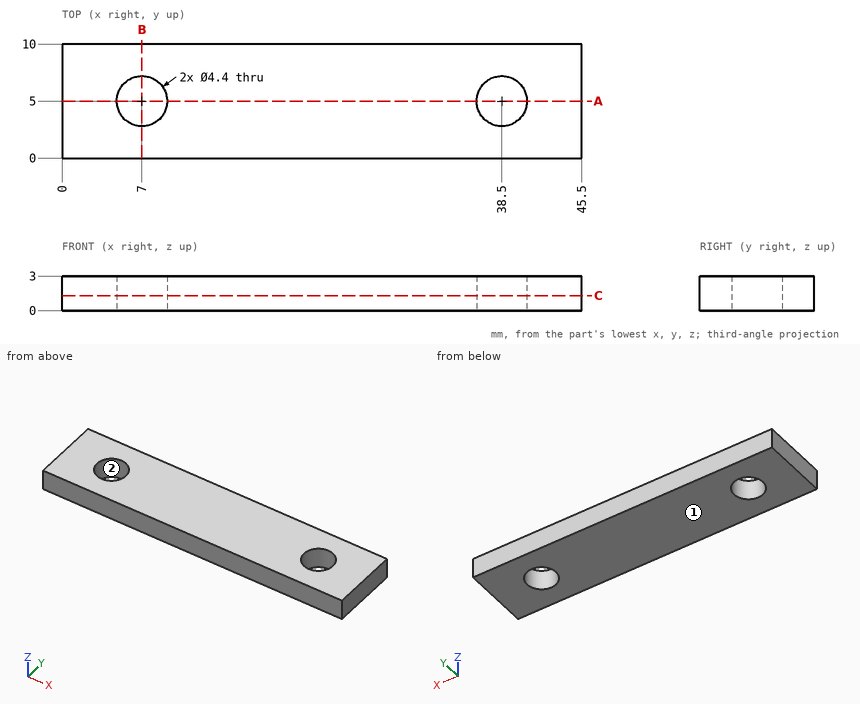
Job drawing, mm, ordinate dimensions from the low corner. One solid piece. Round coordinates to 2 decimals unless told otherwise and drop trailing zeros. Order: outer loops, then holes, each group sorted by start corner. A loop starts at its lowest first (then second) coordinate and runs counter-clockwise, first axis right, second up. Notation, with made-up numbers: (62, 44.25) -> (83, 44.25) arc R35 cw to (83, 78.25) -> close; hole circle Ø2 at (24, -10). An arc over 180 degrees is marked (long way). Write item = value, one per line.
(1) Cut at A-A (y = 5). Write the cut outline in (x, z).
Answers follow:
outline = (0, 0) -> (4.8, 0) -> (4.8, 3) -> (0, 3) -> close; (9.2, 0) -> (36.3, 0) -> (36.3, 3) -> (9.2, 3) -> close; (40.7, 0) -> (45.5, 0) -> (45.5, 3) -> (40.7, 3) -> close
(2) Drill centre lines: L1, parallel to X at y = 5, z = 1.5; L2, parallel to X at y = 7, z = 1.2; L3, parallel to Y at x = 7, z = 2.3. Where is each one in solid material? Low to high.
Answers follow:
L1 = 0 to 4.8, 9.2 to 36.3, 40.7 to 45.5
L2 = 0 to 6.08, 7.92 to 37.58, 39.42 to 45.5
L3 = 0 to 2.8, 7.2 to 10
(3) Pull direction X, two halves, no side cores. Call the marked faces 1 and 2: +X half, -X half, draft (parallel to the pull), parting line (faces both ways), or undercut.
Answers follow:
face_1 = draft
face_2 = undercut
(4) Cut at B-B (x = 7). Write the cut outline in (y, z), plus the area to 3 significant figures.
Answers follow:
outline = (0, 0) -> (2.8, 0) -> (2.8, 3) -> (0, 3) -> close; (7.2, 0) -> (10, 0) -> (10, 3) -> (7.2, 3) -> close
area = 16.8 mm²
(5) Flat gauge pin, fed straight in: P1, Ø3.5, axis at x = 7, y = 5, coming from the +Z side. Where does the tip first touch, or does it go through?
Answers follow:
P1 = through
(6) Cut at C-C (z = 1.3). Write the cut outline in (x, y).
Answers follow:
outline = (0, 0) -> (45.5, 0) -> (45.5, 10) -> (0, 10) -> close; hole circle Ø4.4 at (7, 5); hole circle Ø4.4 at (38.5, 5)
